Geometry: see drawing. Coordinates: mm, zero at the bounding-box minimum. Round coordinates to 2 decimals unless told otherwise and drop trailing zeros. Write each loop counter-clockwise with the first axis right and the second up, starting at its lowest first coordinate (ties: lowest second). Pieces come first, ordered by that corner, then holes. Notation, with made-up numbers: (15, 21) - (24, 21) arc R7 cw to (24, 26) - close; hole circle Ø11 at (-21, 18.5). An arc over 180 degrees is marked (long way). One line per item, written item: value. Start each with the question number.
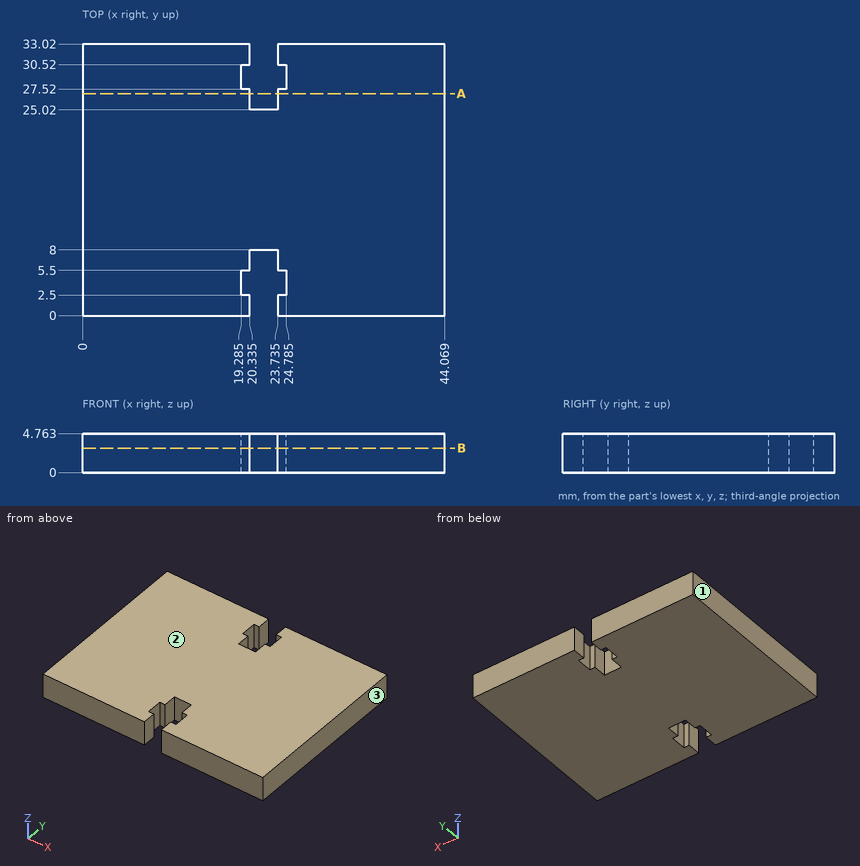
Q1. Cut plane B-B, the plane z = 3. Output: boundary loops of the cut face in (x, y) (1 decimal), and give its area (3 significant figures).
Q2. Pull-direction query (X, two-part tool) for the marked faces 1, 2 and 3; classes: pulls with the +X half, pulls with the -X half, needs draft (parallel to the pull), parting line crosses it, or undercut.
Q3. Material intervals for probe 1 along X at (y, z) = (31, 1.9) (1 decimal); probe 2 along X at (y, z) = (4, 1.6) (1 decimal); probe 3 along Y at (x, z) = (21, 0.55), sorted ascending. Write a range as from..to.
Q4. Cut plane A-A, the plane y = 27. Output: boundary loops of the cut face in (x, z) (1 decimal).
A:
1. outline: (0, 0) - (20.3, 0) - (20.3, 2.5) - (19.3, 2.5) - (19.3, 5.5) - (20.3, 5.5) - (20.3, 8) - (23.7, 8) - (23.7, 5.5) - (24.8, 5.5) - (24.8, 2.5) - (23.7, 2.5) - (23.7, 0) - (44.1, 0) - (44.1, 33) - (23.7, 33) - (23.7, 30.5) - (24.8, 30.5) - (24.8, 27.5) - (23.7, 27.5) - (23.7, 25) - (20.3, 25) - (20.3, 27.5) - (19.3, 27.5) - (19.3, 30.5) - (20.3, 30.5) - (20.3, 33) - (0, 33) - close
1. area: 1,390 mm²
2. face 1: pulls with the -X half
2. face 2: needs draft
2. face 3: pulls with the +X half
3. probe 1: x = 0..20.3, 23.7..44.1
3. probe 2: x = 0..19.3, 24.8..44.1
3. probe 3: y = 8..25.02
4. outline: (0, 0) - (20.3, 0) - (20.3, 4.8) - (0, 4.8) - close; (23.7, 0) - (44.1, 0) - (44.1, 4.8) - (23.7, 4.8) - close
